Could you check a few things on this model? Use its own coordinates, in mm. Face numbers are marked on the shaded views. A direction names the side the tool comes from. Round coordinates to 2 decimals unless told otherwise and drop trailing zeros. Loops run counter-clockwise (first coordinate to the right, second up) from the corner with the lowest first, then second, coordinate; pieces in that order, holes last. Notation, with made-up numbers: (-14.75, 22) -> (43.25, 22) arc R15 ccw to (43.25, 31) -> close; hole circle Ø9 at (45.25, 29.25). An arc over 180 degrees is marked (long way). Put each result on its own line as item: value. Start each with the question number.
1. Which directions (+Z, -Z, +X, -X, +Y, -Y) give clear straight access to the entire face, cutting with the end or side of a thin tool? Please do the marked faces 5, 6, 7 and 8.
2. Imagine slicing it at D-D, the plane y = -20.5. Please give me the cut outline in (x, z).
3. If we mould it in two halves opening along X, with no side actions, what happens to the marked faces 1, 2, 3 and 4? For each: pulls with the +X half, pulls with the -X half, needs draft (parallel to the pull), parting line crosses it, or undercut.
4. I'm going to push flat-ended pins straight in: P1, Ø6, axis at x = -7, z = 8, coming from the +Y side; P2, Ø1.5, axis at y = -11, z = 4.5, coming from the +X side; P3, Ø5, axis at y = -6, z = 10.5, coming from the +X side. Where does each tip first touch, or does it pass through?
5. Imagine slicing it at C-C, the plane z = 15.5. Please give me the cut outline in (x, y), and give its area (3 significant figures).
6. Imagine slicing it at A-A, the plane y = 0. Please give me the cut outline in (x, z).
7. I need wall thicknesses on line 1 (Z direction, x = -5, y = -37); line 2 (X direction, y = 0, z = 12.5); line 3 (X direction, y = -31, z = 8.25). Which ranges of each line are inside material? Lowest first, please. Write a range as [from, to].
8. Imagine slicing it at B-B, the plane x = 0. Please give me the cut outline in (y, z).
```python
from build123d import *

# Parameters (mm, degrees)
BOSS_EXTRUDE1_DEPTH     = 23
FILLET1_R               = 10
CHAMFER1_SIZE           = 0.5
CUT_EXTRUDE1_REACH      = 62.864
CUT_EXTRUDE1_END_RADIUS = 13.25
SKETCH2_W               = 13
SKETCH2_H               = 13
CHAMFER2_SIZE           = 1
CHAMFER3_SIZE           = 0.5


with BuildPart() as part:
    # Sketch1 → Boss-Extrude1 (new body)
    with BuildSketch(Plane.XY):
        with BuildLine():
            Line((-11.5, -14.491376746), (-11.5, -44.491376746))
            Line((-11.5, -44.491376746), (11.5, -44.491376746))
            Line((11.5, -44.491376746), (11.5, -14.491376746))
            ThreePointArc((11.5, -14.491376746), (17.862669336, -4.814046549), (17.224619009, 6.75))
            ThreePointArc((17.224619009, 6.75), (14.31318663, 8.736071822), (11.401754251, 6.75))
            ThreePointArc((11.401754251, 6.75), (0, -13.25), (-11.401754251, 6.75))
            ThreePointArc((-11.401754251, 6.75), (-14.31318663, 8.736071822), (-17.224619009, 6.75))
            ThreePointArc((-17.224619009, 6.75), (-17.862669336, -4.814046549), (-11.5, -14.491376746))
        make_face()
    extrude(amount=BOSS_EXTRUDE1_DEPTH)

    # Fillet1
    fillet1_edges = [part.edges().sort_by_distance(p)[0] for p in [
        (-11.5, -14.491376746, 11.5),
        (11.5, -14.491376746, 11.5),
    ]]
    fillet(fillet1_edges, radius=FILLET1_R)

    # Chamfer1
    chamfer1_edges = [part.edges().sort_by_distance(p)[0] for p in [
        (0, -13.25, 0),
        (14.31318663, 8.736071822, 0),
        (11.5, -31.59983184, 0),
        (14.31318663, 8.736071822, 23),
        (0, -13.25, 23),
        (-14.31318663, 8.736071822, 23),
        (-18.229248977, -3.153487233, 23),
        (-11.5, -31.59983184, 0),
        (-11.5, -31.59983184, 23),
        (18.229248977, -3.153487233, 0),
        (18.229248977, -3.153487233, 23),
        (-12.134141884, -15.203903714, 0),
        (-12.134141884, -15.203903714, 23),
        (12.134141884, -15.203903714, 0),
        (12.134141884, -15.203903714, 23),
        (0, -44.491376746, 23),
        (11.5, -31.59983184, 23),
        (0, -44.491376746, 0),
        (-18.229248977, -3.153487233, 0),
        (-14.31318663, 8.736071822, 0),
    ]]
    chamfer(chamfer1_edges, length=CHAMFER1_SIZE)

    # Cut-Extrude1: up to this cylinder (the profile starts outside it)
    cut_extrude1_end = Plane(origin=(0, 0, 11.5), z_dir=(0, 0, -1)) * Cylinder(CUT_EXTRUDE1_END_RADIUS, 153.228, mode=Mode.PRIVATE)
    # Sketch2 → Cut-Extrude1 (cut, up to the surface)
    with BuildSketch(Plane.XZ.offset(44.491376746), mode=Mode.PRIVATE) as cut_extrude1_sk1:
        with Locations((0, 11.5)):
            Rectangle(SKETCH2_W, SKETCH2_H)
    cut_extrude1_tool1 = extrude(cut_extrude1_sk1.sketch, amount=-CUT_EXTRUDE1_REACH, mode=Mode.PRIVATE) - cut_extrude1_end
    add(cut_extrude1_tool1.solids().sort_by_distance((0, -44.491377, 11.5))[0], mode=Mode.SUBTRACT)

    # Chamfer2
    chamfer2_edges = [part.edges().sort_by_distance(p)[0] for p in [
        (-6.5, -28.018739992, 5),
        (-6.5, -28.018739992, 18),
        (6.5, -28.018739992, 18),
        (6.5, -28.018739992, 5),
    ]]
    chamfer(chamfer2_edges, length=CHAMFER2_SIZE)

    # Chamfer3
    chamfer3_edges = [part.edges().sort_by_distance(p)[0] for p in [
        (0, -44.491376746, 5),
        (-6.5, -44.491376746, 11.5),
        (6.5, -44.491376746, 11.5),
        (0, -44.491376746, 18),
        (-6, -44.491376746, 5.5),
        (6, -44.491376746, 5.5),
        (6, -44.491376746, 17.5),
        (-6, -44.491376746, 17.5),
        (-11.5, -44.491376746, 11.5),
        (11.5, -44.491376746, 11.5),
    ]]
    chamfer(chamfer3_edges, length=CHAMFER3_SIZE)


solid = part.part
```
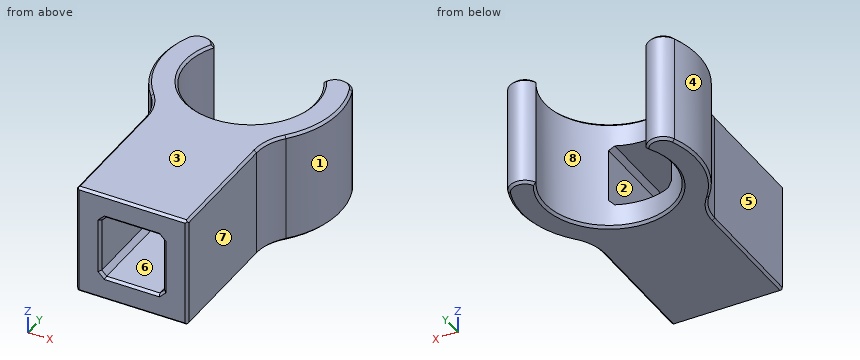
Entries:
1. face 5: +Z, -Z, -X, -Y
1. face 6: +Y, -Y
1. face 7: +Z, -Z, +X, -Y
1. face 8: +Z, -Z
2. outline: (-11.5, 0.5) -> (-11, 0) -> (11, 0) -> (11.5, 0.5) -> (11.5, 22.5) -> (11, 23) -> (-11, 23) -> (-11.5, 22.5) -> close; hole (-6.5, 6) -> (-5.5, 5) -> (5.5, 5) -> (6.5, 6) -> (6.5, 17) -> (5.5, 18) -> (-5.5, 18) -> (-6.5, 17) -> close
3. face 1: pulls with the +X half
3. face 2: undercut
3. face 3: needs draft
3. face 4: pulls with the -X half
4. P1: y = -8.69
4. P2: x = 15.4
4. P3: x = 18.17
5. outline: (-17.22, 6.75) arc R18.5 ccw to (-13.96, -12.14) arc R10 cw to (-11.5, -18.71) -> (-11.5, -43.99) -> (-11, -44.49) -> (-7, -44.49) -> (-6.5, -43.99) -> (-6.5, -11.55) arc R13.25 cw to (-11.4, 6.75) arc R3.13 ccw to start; (6.5, -43.99) -> (7, -44.49) -> (11, -44.49) -> (11.5, -43.99) -> (11.5, -18.71) arc R10 cw to (13.96, -12.14) arc R18.5 ccw to (17.22, 6.75) arc R3.13 ccw to (11.4, 6.75) arc R13.25 cw to (6.5, -11.55) -> close
5. area: 569 mm^2
6. outline: (-18.5, 0.5) -> (-18, 0) -> (-13.75, 0) -> (-13.25, 0.5) -> (-13.25, 22.5) -> (-13.75, 23) -> (-18, 23) -> (-18.5, 22.5) -> close; (13.25, 0.5) -> (13.75, 0) -> (18, 0) -> (18.5, 0.5) -> (18.5, 22.5) -> (18, 23) -> (13.75, 23) -> (13.25, 22.5) -> close
7. line 1: [0, 5], [18, 23]
7. line 2: [-18.5, -13.25], [13.25, 18.5]
7. line 3: [-11.5, -6.5], [6.5, 11.5]
8. outline: (-44.49, 0.5) -> (-43.99, 0) -> (-13.75, 0) -> (-13.25, 0.5) -> (-13.25, 5) -> (-43.99, 5) -> (-44.49, 4.5) -> close; (-44.49, 18.5) -> (-43.99, 18) -> (-13.25, 18) -> (-13.25, 22.5) -> (-13.75, 23) -> (-43.99, 23) -> (-44.49, 22.5) -> close
